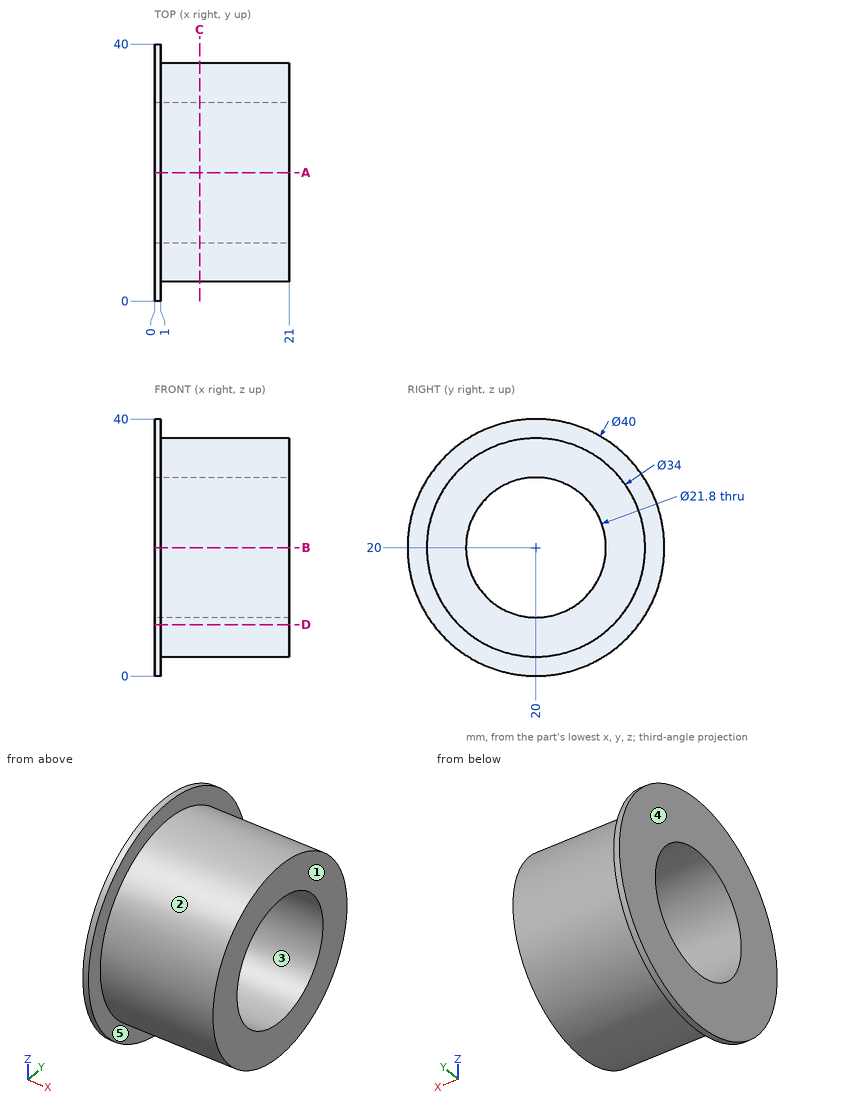
Can you work these out from the drawing? Everything is in mm from the part's minimum corner. A direction names the side the tool comes from. Round coordinates to 2 decimals unless told otherwise and drop trailing zeros. Write each loop counter-clockwise with the first axis right and the second up, starting at its lowest first coordinate (ties: lowest second). Pieces come first, ordered by that corner, then holes. Notation, with made-up numbers: M 89.25,-11 L 111.25,-11 A21 cw 111.25,7 Z; hole C 54,58 d9. An arc over 180 degrees is marked long. Use a Markdown table: item, result.
Item 1: I want a section at D-D (z = 8). List the corners of the cut face in (x, y) for me, and give its area (3 significant figures).
Found:
| item | result |
|---|---|
| outline | M 0,4 L 1,4 L 1,7.96 L 21,7.96 L 21,32.04 L 1,32.04 L 1,36 L 0,36 Z |
| area | 514 mm2 |
Item 2: Which directions (+Z, -Z, +X, -X, +Y, -Y) give clear straight access to the entire face, cutting with the end or side of a thin tool? Please do the marked faces 4 and 5.
Found:
| item | result |
|---|---|
| face 4 | +Z, -Z, -X, +Y, -Y |
| face 5 | +X |
Item 3: We'd pull the mould along Y, two halves only. Please class the marked faces 1, 2 and 3: released by +Y, released by -Y, zero draft, split by the parting line, or undercut.
Found:
| item | result |
|---|---|
| face 1 | zero draft |
| face 2 | split by the parting line |
| face 3 | undercut |
Item 4: I want a section at A-A (y = 20). List the corners of the cut face in (x, z) for me, and give its area (3 significant figures).
Found:
| item | result |
|---|---|
| outline | M 0,0 L 1,0 L 1,3 L 21,3 L 21,9.1 L 0,9.1 Z; M 0,30.9 L 21,30.9 L 21,37 L 1,37 L 1,40 L 0,40 Z |
| area | 262 mm2 |
Item 5: For pin 1 Ø5 at (x, z) = (15, 22.5) entering from -Y; pin 2 Ø6 at (x, y) = (12, 34.5) entering from +Z; pin 3 Ø10 at (x, y) = (4.5, 26.5) entering from -Z; pin 4 Ø12 at (x, z) = (3.5, 16.5) entering from -Y, each with a flat end and sliding along its axis, tell me the tip position at first contact or that it passes through.
Found:
| item | result |
|---|---|
| pin 1 | stops at y = 3 |
| pin 2 | stops at z = 32.52 |
| pin 3 | stops at z = 0.22 |
| pin 4 | stops at y = 0 |
Item 6: If I drill on line 1 along Y through (x, z) = (6, 20); line 2 along Y through (x, z) = (1.75, 15.5); line 3 along Z through (x, y) = (19, 15), over which ranges is the centre line in solid material (lowest first)? Write a range as [from, to].
Found:
| item | result |
|---|---|
| line 1 | y = [3, 9.1], [30.9, 37] |
| line 2 | y = [3.61, 10.07], [29.93, 36.39] |
| line 3 | z = [3.75, 10.31], [29.69, 36.25] |
Item 7: I want a section at C-C (x = 7). List the corners of the cut face in (y, z) for me, and give its area (3 significant figures).
Found:
| item | result |
|---|---|
| outline | C 20,20 d34; hole C 20,20 d21.8 |
| area | 535 mm2 |
